CAD build for the part. Positions are in the model's coordinates, mm. A direction names the side the tool comes from. Give positions to 0.01 mm unless a question says otherwise; leave off trailing zeros. Answer in a Markdown table with one row per item. Add a question column.
```python
from build123d import *

# Parameters (mm, degrees)
F1_DEPTH = 70


# Not quite as in the source:
# - ends of sketch curves that miss each other by under 0.0002 mm in the source are joined


with BuildPart() as f1:
    # F0 (on Right) → F1 (new body, symmetric)
    with BuildSketch(Plane.YZ):
        with BuildLine():
            Line((9.043565, 10.073321), (0.043565, 10.073321))
            Line((0.043565, 10.073321), (-8.956435, 10.073321))
            ThreePointArc((-8.956435, 10.073321), (-9.6635417812, 9.7804277812), (-9.956435, 9.073321))
            Line((-9.956435, 9.073321), (-9.956435, 3.373321))
            ThreePointArc((-9.956435, 3.373321), (-9.8685670344, 3.1611889656), (-9.656435, 3.073321))
            Line((-9.656435, 3.073321), (-8.256435, 3.073321))
            ThreePointArc((-8.256435, 3.073321), (-8.0443029656, 3.1611889656), (-7.956435, 3.373321))
            Line((-7.956435, 3.373321), (-7.956435, 6.073321))
            Line((-7.956435, 6.073321), (-7.017095, 6.073321))
            Line((-7.017095, 6.073321), (-3.956435, 3.012661))
            Line((-3.956435, 3.012661), (-3.956435, 0.726911))
            ThreePointArc((-3.956435, 0.726911), (-3.9393979324, 0.5975015494), (-3.8894477764, 0.4769111291))
            Line((-3.8894477764, 0.4769111291), (-3.656435, 0.073321))
            Line((-3.656435, 0.073321), (-3.889448, -0.330269))
            ThreePointArc((-3.889448, -0.330269), (-3.956435, -0.580269), (-3.8894477764, -0.8302688709))
            Line((-3.8894477764, -0.8302688709), (-3.707412, -1.145565))
            Line((-3.707412, -1.145565), (-3.956435, -2.426679))
            Line((-3.956435, -2.426679), (-3.956435, -2.866019))
            Line((-3.956435, -2.866019), (-7.017095, -5.926679))
            Line((-7.017095, -5.926679), (-7.956435, -5.926679))
            Line((-7.956435, -5.926679), (-7.956435, -3.226679))
            ThreePointArc((-7.956435, -3.226679), (-8.0443029656, -3.0145469656), (-8.256435, -2.926679))
            Line((-8.256435, -2.926679), (-9.656435, -2.926679))
            ThreePointArc((-9.656435, -2.926679), (-9.8685670344, -3.0145469656), (-9.956435, -3.226679))
            Line((-9.956435, -3.226679), (-9.956435, -8.926679))
            ThreePointArc((-9.956435, -8.926679), (-9.6635417812, -9.6337857812), (-8.956435, -9.926679))
            Line((-8.956435, -9.926679), (-3.256435, -9.926679))
            ThreePointArc((-3.256435, -9.926679), (-3.0443029656, -9.8388110344), (-2.956435, -9.626679))
            Line((-2.956435, -9.626679), (-2.956435, -8.226679))
            ThreePointArc((-2.956435, -8.226679), (-3.0443029656, -8.0145469656), (-3.256435, -7.926679))
            Line((-3.256435, -7.926679), (-5.956435, -7.926679))
            Line((-5.956435, -7.926679), (-5.956435, -6.987339))
            Line((-5.956435, -6.987339), (-2.895775, -3.926679))
            Line((-2.895775, -3.926679), (-0.610025, -3.926679))
            ThreePointArc((-0.610025, -3.926679), (-0.4806155494, -3.9096419324), (-0.3600251291, -3.8596917764))
            Line((-0.3600251291, -3.8596917764), (-0.0645959325, -3.6891257984))
            Line((-0.0645959325, -3.6891257984), (0.2217128734, -3.8544264098))
            ThreePointArc((0.2217128734, -3.8544264098), (0.3921793907, -3.9150473077), (0.5730594828, -3.9110345539))
            ThreePointArc((0.5730594828, -3.9110345539), (0.6346161199, -3.9227524708), (0.697155, -3.926679))
            Line((0.697155, -3.926679), (2.982905, -3.926679))
            Line((2.982905, -3.926679), (6.043565, -6.987339))
            Line((6.043565, -6.987339), (6.043565, -7.926679))
            Line((6.043565, -7.926679), (3.343565, -7.926679))
            ThreePointArc((3.343565, -7.926679), (3.1314329656, -8.0145469656), (3.043565, -8.226679))
            Line((3.043565, -8.226679), (3.043565, -9.626679))
            ThreePointArc((3.043565, -9.626679), (3.1314329656, -9.8388110344), (3.343565, -9.926679))
            Line((3.343565, -9.926679), (9.043565, -9.926679))
            ThreePointArc((9.043565, -9.926679), (9.7506717812, -9.6337857812), (10.043565, -8.926679))
            Line((10.043565, -8.926679), (10.043565, -3.226679))
            ThreePointArc((10.043565, -3.226679), (9.9556970344, -3.0145469656), (9.743565, -2.926679))
            Line((9.743565, -2.926679), (8.343565, -2.926679))
            ThreePointArc((8.343565, -2.926679), (8.1314329656, -3.0145469656), (8.043565, -3.226679))
            Line((8.043565, -3.226679), (8.043565, -5.926679))
            Line((8.043565, -5.926679), (7.104225, -5.926679))
            Line((7.104225, -5.926679), (4.043565, -2.866019))
            Line((4.043565, -2.866019), (4.043565, -2.426679))
            Line((4.043565, -2.426679), (3.794542, -1.145565))
            Line((3.794542, -1.145565), (3.976578, -0.830269))
            ThreePointArc((3.976578, -0.830269), (4.043565, -0.580269), (3.9765777764, -0.3302691291))
            Line((3.9765777764, -0.3302691291), (3.743565, 0.073321))
            Line((3.743565, 0.073321), (3.976578, 0.476911))
            ThreePointArc((3.976578, 0.476911), (4.0265279324, 0.5975015494), (4.043565, 0.726911))
            Line((4.043565, 0.726911), (4.043565, 3.012661))
            Line((4.043565, 3.012661), (7.104225, 6.073321))
            Line((7.104225, 6.073321), (8.043565, 6.073321))
            Line((8.043565, 6.073321), (8.043565, 3.373321))
            ThreePointArc((8.043565, 3.373321), (8.1314329656, 3.1611889656), (8.343565, 3.073321))
            Line((8.343565, 3.073321), (9.743565, 3.073321))
            ThreePointArc((9.743565, 3.073321), (9.9556970344, 3.1611889656), (10.043565, 3.373321))
            Line((10.043565, 3.373321), (10.043565, 9.073321))
            ThreePointArc((10.043565, 9.073321), (9.7506717812, 9.7804277812), (9.043565, 10.073321))
        make_face()
        with BuildLine():
            ThreePointArc((0.043565, 2.173321), (2.143565, 0.073321), (0.043565, -2.026679))
            ThreePointArc((0.043565, -2.026679), (-2.056435, 0.073321), (0.043565, 2.173321))
        make_face(mode=Mode.SUBTRACT)
        with BuildLine():
            Line((2.775798, 4.073321), (0.043565, 4.073321))
            Line((0.043565, 4.073321), (-2.688668, 4.073321))
            ThreePointArc((-2.688668, 4.073321), (-2.8800097162, 4.1113812337), (-3.0422213906, 4.2197676094))
            Line((-3.0422213906, 4.2197676094), (-5.809988, 6.987535))
            ThreePointArc((-5.809988, 6.987535), (-5.9183747663, 7.1497462838), (-5.956435, 7.341088))
            Line((-5.956435, 7.341088), (-5.956435, 7.573321))
            ThreePointArc((-5.956435, 7.573321), (-5.8099883906, 7.9268743906), (-5.456435, 8.073321))
            Line((-5.456435, 8.073321), (0.043565, 8.073321))
            Line((0.043565, 8.073321), (5.543565, 8.073321))
            ThreePointArc((5.543565, 8.073321), (5.8971183906, 7.9268743906), (6.043565, 7.573321))
            Line((6.043565, 7.573321), (6.043565, 7.341088))
            ThreePointArc((6.043565, 7.341088), (6.0055047663, 7.1497462838), (5.8971183906, 6.9875346094))
            Line((5.8971183906, 6.9875346094), (3.129351, 4.219768))
            ThreePointArc((3.129351, 4.219768), (2.9671397162, 4.1113812337), (2.775798, 4.073321))
        make_face(mode=Mode.SUBTRACT)
    extrude(amount=F1_DEPTH, both=True)


solid = f1.part
```
Item 1: Probe L1, parallel to Z at x = 25, y = -1; L2, parallel to Y at x = 2.5, z = -3.75; L3, parallel to Y at x = 59, z = -5. List the from-to ranges inside material, lowest first. Write a range as from..to.
Item 2: Slice it at A-A, the plane x = -19.5. State how many separate pieces and enclosed holes the cut face has, then the cut area to 3 significant figures.
Item 3: Drop flat-ended pins along their axis: pin 1 Ø2.5 at (y, z) = (0.04, 0.07) entering from +X; pin 2 Ø1.1 at (x, z) = (-30.5, 1.5) entering from +Y; pin 3 Ø0.7 at (x, z) = (23, 1.5) entering from -Y; pin 4 Ø1 at (x, y) = (24.5, 0) entering from -Z. Give the stop position or say it passes through.
Item 4: Mould opens along Y. For faces 5 (the face through (1, -9.956, -6)), 6 (the face through (70, -0.1, 2.4)), 7 (the face through (1, 5, -7.927)), 8 (the face through (0.98, -5.465, -4.375)) say: released by +Y, released by -Y, zero draft, split by the parting line, or undercut.
Item 5: Which spindle directions (+Z, -Z, +X, -X, +Y, -Y) get a long thin tool onto all of the face, cutting with end or side? Do faces 1 (the face through (1, 2, -3.927)), 2 (the face through (1, -5, -7.927)), 3 (the face through (1, 10.044, 6)), 4 (the face through (1, 4.044, 2)). Say none if no direction does.
Answer key:
| question | item | result |
|---|---|---|
| 1 | L1 | z = -3.93..-1.75, 1.9..4.07, 8.07..10.07 |
| 1 | L2 | y = -9.96..-7.96, -4.84..-0.17, 0.04..4.93, 8.04..10.04 |
| 1 | L3 | y = -9.96..-7.96, -6.09..-3.97, 4.06..6.18, 8.04..10.04 |
| 2 | separate pieces | 1 |
| 2 | enclosed holes | 2 |
| 2 | area | 194 mm² |
| 3 | pin 1 | passes through |
| 3 | pin 2 | stops at y = 4.04 |
| 3 | pin 3 | stops at y = -3.96 |
| 3 | pin 4 | stops at z = -3.92 |
| 4 | face 5 | released by -Y |
| 4 | face 6 | zero draft |
| 4 | face 7 | undercut |
| 4 | face 8 | undercut |
| 5 | face 1 | -Z, +X, -X |
| 5 | face 2 | +X, -X |
| 5 | face 3 | +Z, -Z, +X, -X, +Y |
| 5 | face 4 | +X, -X, +Y |
